Here's how the part is built. I have some questions about the finished solid (model axes, mm). Face numbers are marked on the shaded views. A direction names the side the tool comes from. Round coordinates to 2 decimals unless told otherwise and drop trailing zeros. Write each loop counter-clockwise with the first axis right and the second up, starting at its lowest first coordinate (ties: lowest second). Pieces come first, ordered by that corner, then holes. Notation, with made-up numbers: M 87.25,24.25 L 135.25,24.25 A24 cw 135.25,49.25 Z; hole C 20.25,-8.75 d8. An arc over 180 degrees is marked long. Use a Markdown table: item, result. Add a question column.
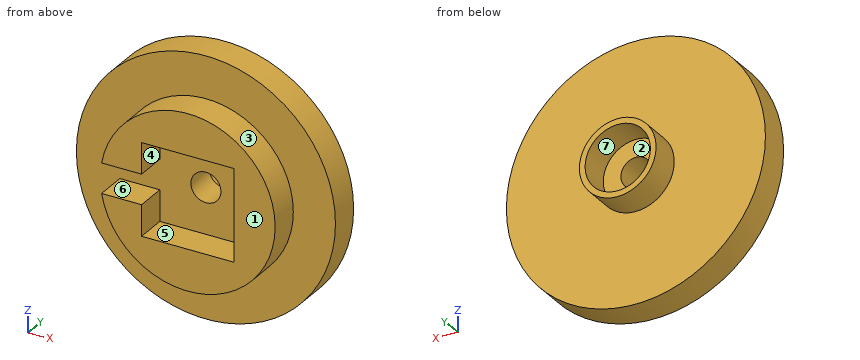
Autodesk Inventor part; units mm, degrees
ref_plane "YZ Plane" through (0, 0, 0) normal (1, 0, 0) x (0, 1, 0)
ref_plane "XZ Plane" through (0, 0, 0) normal (0, 1, 0) x (-1, 0, 0)
ref_plane "XY Plane" through (0, 0, 0) normal (0, 0, 1) x (1, 0, 0)
sketch "Sketch1" plane through (0, 0, 0) normal (0, 1, 0) x (-1, 0, 0)
  circle A0 centre (0, 0) radius 12.5
  circle A1 centre (0, 0) radius 1.45
  dimension "d0" = 25
  dimension "d1" = 2.9
extrude "Extrusion1" add sketch "Sketch1" along normal blind 3
sketch "Sketch2" plane through (0, 3, 0) normal (0, 1, 0) x (1, 0, 0)
  circle A0 centre (0, 0) radius 1.45
  circle A1 centre (0, 0) radius 3.15
  circle A2 centre (0, 0) radius 3.7
  dimension "d4" = 6.3
  dimension "d5" = 7.4
extrude "Extrusion2" add sketch "Sketch2" along normal blind 3 contours A2
sketch "Sketch3" plane through (0, 0, 0) normal (0, -1, 0) x (1, 0, 0)
  circle A0 centre (0, 0) radius 1.45
  line L0 (-4.45, -4.45) -> (4.45, -4.45)
  line L1 (4.45, -4.45) -> (4.45, 4.45)
  line L2 (4.45, 4.45) -> (-4.45, 4.45)
  line L3 (-4.45, 4.45) -> (-4.45, -4.45)
  line L4 (-4.45, -4.45) -> (4.45, 4.45) construction
  line L5 (4.45, -4.45) -> (-4.45, 4.45) construction
  circle A1 centre (0, 0) radius 8.4362
  line L6 (-4.45, 1.45) -> (-8.3107, 1.45)
  line L7 (-4.45, -1.45) -> (-8.3107, -1.45)
  dimension "d8" = 8.9
  dimension "d9" = 8.9
extrude "Extrusion3" add sketch "Sketch3" along normal blind 3 contours L0 L1 L2 L3 L6 A1 L7
properties part number "30_CUBE_openSIM_Laser_FPC_mount"
Item 1: Imagine slicing it at B-B on z = 0. List the corners of the cut face in (x, y) for me, plus the area to 3 significant figures.
Item 2: Imagine slicing it at A-A on x = 0. List the corners of the cut face in (y, z) for me, plus the area to 3 significant figures.
Item 3: Imagine slicing it at D-D on x = -6. List the corners of the cut face in (y, z) for me.
Item 4: For pin 1 Ø5 at (x, y) = (1.5, 4.5) entering from -Z; pin 2 Ø0.9 at (x, y) = (-6.5, -1) entering from +Z; pin 3 Ø2.5 at (y, z) = (-1, 1) entering from -X; pin 4 Ø1.5 at (y, z) = (-0.5, -8) entering from -X, each with a flat end and sliding along its axis, tell me the tip position at first contact or that it passes through.
Item 5: I need wall thicknesses on probe 1 along Z at (x, y) = (0, 3.85); probe 2 along Z at (x, y) = (0, 1.3). Which ranges of each line are inside material? Lowest first, please. Write a range as from..to.
Item 6: Imagine slicing it at C-C on y = 0.5. List the corners of the cut face in (x, z) for me.
Item 7: On a 3-axis mill with a long thin cutter (end or side, diameter ignored), from which of +Z, -Z, +X, -X, +Y, -Y can I reach the whole of each face in a straight line? I mean the marked faces 5, 6 and 7. Say none if no direction works.
Item 8: If we mould it in two halves opening along X, with no side actions, what happens to the marked faces 1, 2, 3 and 4? For each: +X half, -X half, draft (parallel to the pull), parting line (faces both ways), or undercut.
The answers:
| question | item | result |
|---|---|---|
| 1 | outline | M -12.5,0 L -1.45,0 L -1.45,3 L -3.15,3 L -3.15,6 L -3.7,6 L -3.7,3 L -12.5,3 Z; M 1.45,0 L 4.45,0 L 4.45,-3 L 8.44,-3 L 8.44,0 L 12.5,0 L 12.5,3 L 3.7,3 L 3.7,6 L 3.15,6 L 3.15,3 L 1.45,3 Z |
| 1 | area | 81.6 mm² |
| 2 | outline | M -3,-8.44 L 0,-8.44 L 0,-12.5 L 3,-12.5 L 3,-3.7 L 6,-3.7 L 6,-3.15 L 3,-3.15 L 3,-1.45 L 0,-1.45 L 0,-4.45 L -3,-4.45 Z; M -3,4.45 L 0,4.45 L 0,1.45 L 3,1.45 L 3,3.15 L 6,3.15 L 6,3.7 L 3,3.7 L 3,12.5 L 0,12.5 L 0,8.44 L -3,8.44 Z |
| 2 | area | 93.5 mm² |
| 3 | outline | M -3,-5.93 L 0,-5.93 L 0,-10.97 L 3,-10.97 L 3,10.97 L 0,10.97 L 0,5.93 L -3,5.93 L -3,1.45 L 0,1.45 L 0,-1.45 L -3,-1.45 Z |
| 4 | pin 1 | z = -12.5 |
| 4 | pin 2 | z = 5.88 |
| 4 | pin 3 | x = -12.5 |
| 4 | pin 4 | x = -10.04 |
| 5 | probe 1 | -3.7..-3.15, 3.15..3.7 |
| 5 | probe 2 | -12.5..-1.45, 1.45..12.5 |
| 6 | outline | C 0,0 d25; hole C 0,0 d2.9 |
| 7 | face 5 | -Y |
| 7 | face 6 | -X, -Y |
| 7 | face 7 | +Y |
| 8 | face 1 | draft |
| 8 | face 2 | undercut |
| 8 | face 3 | parting line |
| 8 | face 4 | undercut |
